from build123d import *

# Parameters (mm, degrees)
SKETCH1_W           = 78.2
SKETCH1_H           = 78.2
SKETCH1_W_2         = 60.2
SKETCH1_H_2         = 60.2
BOSS_EXTRUDE1_DEPTH = 40
SKETCH2_W           = 78.2
SKETCH2_H           = 78.2
SKETCH2_R           = 2
BOSS_EXTRUDE2_DEPTH = 3
SKETCH3_W           = 15.098438038
SKETCH3_H           = 4
CUT_EXTRUDE1_DEPTH  = 19
SKETCH4_R           = 4.1
CUT_EXTRUDE2_DEPTH  = 1.1
SKETCH5_W           = 30
SKETCH5_H           = 5
BOSS_EXTRUDE3_DEPTH = 5


with BuildPart() as part:
    # Sketch1 → Boss-Extrude1 (new body)
    with BuildSketch(Plane(origin=(0, 0, 0), x_dir=(0, 0, -1), z_dir=(1, 0, 0))):
        Rectangle(SKETCH1_W, SKETCH1_H)
        Rectangle(SKETCH1_W_2, SKETCH1_H_2, mode=Mode.SUBTRACT)
    extrude(amount=BOSS_EXTRUDE1_DEPTH)

    # Sketch2 → Boss-Extrude2 (add)
    # profile 1 of 6: a face of its own
    with BuildSketch(Plane(origin=(40, 0, 0), x_dir=(0, 0, -1), z_dir=(1, 0, 0))):
        Rectangle(SKETCH2_W, SKETCH2_H)
        Polygon((-30.1, 15.1), (-30.1, 30.1), (-15.1, 30.1), (15.1, 30.1), (30.1, 30.1), (30.1, 15.1), (30.1, -15.1), (30.1, -30.1), (15.1, -30.1), (-15.1, -30.1), (-30.1, -30.1), (-30.1, -15.1), align=None, mode=Mode.SUBTRACT)
    # profile 2 of 6: a face of its own
    with BuildSketch(Plane(origin=(40, 0, 0), x_dir=(0, 0, -1), z_dir=(1, 0, 0))):
        Polygon((-15.1, -30.1), (-30.1, -15.1), (-30.1, -30.1), align=None)
        with Locations((-26.135533906, -26.135533906)):
            Circle(SKETCH2_R, mode=Mode.SUBTRACT)
    # profile 3 of 6: a face of its own
    with BuildSketch(Plane(origin=(40, 0, 0), x_dir=(0, 0, -1), z_dir=(1, 0, 0))):
        Polygon((30.1, -15.1), (15.1, -30.1), (30.1, -30.1), align=None)
        with Locations((26.135533906, -26.135533906)):
            Circle(SKETCH2_R, mode=Mode.SUBTRACT)
    # profile 4 of 6: a face of its own
    with BuildSketch(Plane(origin=(40, 0, 0), x_dir=(0, 0, -1), z_dir=(1, 0, 0))):
        Polygon((30.1, 30.1), (15.1, 30.1), (30.1, 15.1), align=None)
        with Locations((26.135533906, 26.135533906)):
            Circle(SKETCH2_R, mode=Mode.SUBTRACT)
    # profile 5 of 6: a face of its own
    with BuildSketch(Plane(origin=(40, 0, 0), x_dir=(0, 0, -1), z_dir=(1, 0, 0))):
        with BuildLine():
            Line((-15.1, 30.1), (-30.1, 30.1))
            Line((-30.1, 30.1), (-27.549747468, 27.549747468))
            ThreePointArc((-27.549747468, 27.549747468), (-25.370167041, 27.983292971), (-24.135533906, 26.135533906))
            ThreePointArc((-24.135533906, 26.135533906), (-24.287774841, 25.370167041), (-24.721320344, 24.721320344))
            Line((-24.721320344, 24.721320344), (-22.6, 22.6))
            Line((-22.6, 22.6), (-15.1, 30.1))
        make_face()
    # profile 6 of 6: a face of its own
    with BuildSketch(Plane(origin=(40, 0, 0), x_dir=(0, 0, -1), z_dir=(1, 0, 0))):
        with BuildLine():
            Line((-27.549747468, 27.549747468), (-30.1, 30.1))
            Line((-30.1, 30.1), (-30.1, 15.1))
            Line((-30.1, 15.1), (-22.6, 22.6))
            Line((-22.6, 22.6), (-24.721320344, 24.721320344))
            ThreePointArc((-24.721320344, 24.721320344), (-27.549747468, 24.721320344), (-27.549747468, 27.549747468))
        make_face()
    extrude(amount=BOSS_EXTRUDE2_DEPTH)

    # Sketch3 → Cut-Extrude1 (cut, symmetric)
    with BuildSketch(Plane(origin=(0, -30.1, 0), x_dir=(1, 0, 0), z_dir=(0, 1, 0))):
        with Locations((43, -14.215479316)):
            Rectangle(SKETCH3_W, SKETCH3_H)
    extrude(amount=CUT_EXTRUDE1_DEPTH, both=True, mode=Mode.SUBTRACT)

    # Sketch4 → Cut-Extrude2 (cut, symmetric)
    with BuildSketch(Plane.ZY):
        with Locations((-34.6, 34.6)):
            Circle(SKETCH4_R)
        with Locations((-34.6, -34.6)):
            Circle(SKETCH4_R)
        with Locations((34.6, -34.6)):
            Circle(SKETCH4_R)
        with BuildLine():
            ThreePointArc((37.499137803, 37.499137803), (31.700862197, 37.499137803), (31.700862197, 31.700862197))
            Line((31.700862197, 31.700862197), (37.499137803, 37.499137803))
        make_face()
        with BuildLine():
            Line((37.499137803, 37.499137803), (31.700862197, 31.700862197))
            ThreePointArc((31.700862197, 31.700862197), (36.169002073, 30.812093917), (38.7, 34.6))
            ThreePointArc((38.7, 34.6), (38.387906083, 36.169002073), (37.499137803, 37.499137803))
        make_face()
    extrude(amount=CUT_EXTRUDE2_DEPTH, both=True, mode=Mode.SUBTRACT)

    # Sketch5 → Boss-Extrude3 (add)
    with BuildSketch(Plane.XZ.offset(39.1)):
        with Locations((28, -26.6)):
            Rectangle(SKETCH5_W, SKETCH5_H)
        with Locations((28, 26.6)):
            Rectangle(SKETCH5_W, SKETCH5_H)
    extrude(amount=BOSS_EXTRUDE3_DEPTH)


solid = part.part
For this review, take the finished solid that the model builds, in its own axes (mm). A direction names the side the tool comes from. Give positions to 0.01 mm unless a question says otherwise; leave off trailing zeros. Write each loop counter-clockwise with the first axis right and the second up, starting at its lowest first coordinate (ties: lowest second). Pieces come first, ordered by that corner, then holes. Notation, with made-up numbers: (43, 14.5) -> (83, 14.5) arc R17 ccw to (83, 34.5) -> close; hole circle Ø9 at (84, -31.75). An arc over 180 degrees is marked (long way). Use CSV: the item, a comma, the result in double quotes.
Q1. Take a section at B-B, the plane z = 17.5. Write out the cut boundary in (x, y), then the cut area to 3 significant figures.
Conclusion:
outline,"(0, -39.1) -> (43, -39.1) -> (43, -27.7) -> (40, -27.7) -> (40, -30.1) -> (0, -30.1) -> close; (0, 30.1) -> (40, 30.1) -> (40, 27.7) -> (43, 27.7) -> (43, 39.1) -> (0, 39.1) -> close"
area,"788 mm2"
Q2. Mouldability with a two-part tool opening along Z and no side actions: class faces 1 (the face through (28, -42, -29.1)), 2 (the face through (13, -42, 27)), 3 (the face through (1.1, 35, -35)) as pulls with the +Z half, pulls with the -Z half, needs draft (parallel to the pull), parting line crosses it, or undercut.
Conclusion:
face 1,"pulls with the -Z half"
face 2,"needs draft"
face 3,"undercut"
Q3. To check wall thickness, follow probe 1 along Y at (x, z) = (0.95, 34.6); probe 2 along Y at (x, z) = (19.5, -16.5). State the ranges of each line that lie inside material, in increasing order. Write a range as [from, to].
Conclusion:
probe 1,"[-39.1, -38.7], [-30.5, 30.5], [38.7, 39.1]"
probe 2,"[-39.1, -30.1], [30.1, 39.1]"
Q4. Take a section at D-D, the plane z = 34.6. Write out the cut boundary in (x, y), then the cut area to 3 significant figures.
Conclusion:
outline,"(0, -39.1) -> (43, -39.1) -> (43, 39.1) -> (0, 39.1) -> (0, 38.7) -> (1.1, 38.7) -> (1.1, 30.5) -> (0, 30.5) -> (0, -30.5) -> (1.1, -30.5) -> (1.1, -38.7) -> (0, -38.7) -> close"
area,"3,340 mm2"
Q5. Take a section at C-C, the plane x = 11. Write out the cut boundary in (y, z).
Conclusion:
outline,"(-39.1, -39.1) -> (39.1, -39.1) -> (39.1, 39.1) -> (-39.1, 39.1) -> close; hole (-30.1, -30.1) -> (30.1, -30.1) -> (30.1, 30.1) -> (-30.1, 30.1) -> close"
Q6. For P1, Ø7.5, axis at y = 23.5, z = -21, coming from the -X side; P2, Ø12, axis at y = -22, z = -24.5, coming from the -X side; P3, Ø2, axis at y = -36.5, z = 15, coming from the +X side; P4, Ø2.5, axis at y = -35, z = 33, coming from the -X side, all flat-tipped, find the tip position at first contact; note any pin that passes through.
Conclusion:
P1,"x = 40"
P2,"x = 0"
P3,"x = 35.45"
P4,"x = 1.1"
Q7. Tool access review of faces 4 (the face through (35.451, -35, 14)), 5 (the face through (41.5, -22.1, 23.1)), 6 (the face through (40, -24, -24)), 7 (the face through (28, -42, -24.1)): name each direction out of +Z, -Z, +X, -X, +Y, -Y from which nothing blocks a thin tool from reaching the whole face with its end or side.
Conclusion:
face 4,"+X, -Y"
face 5,"+X, -X"
face 6,"-X"
face 7,"+X, -X, -Y"
Q8. Take a section at A-A, the plane y = 7.5. Write out the cut boundary in (x, z), then the cut area to 3 significant figures.
Conclusion:
outline,"(0, -39.1) -> (43, -39.1) -> (43, -30.1) -> (0, -30.1) -> close; (0, 30.1) -> (43, 30.1) -> (43, 39.1) -> (0, 39.1) -> close"
area,"774 mm2"
